from build123d import *

# Parameters (mm, degrees)
ESQUISSE1_W             = 30.5
ESQUISSE1_H             = 30.5
BOSS_EXTRU_1_DEPTH      = 9.35
TROU_TARAUD_M31_D       = 2.5
TROU_TARAUD_M31_DEPTH   = 8.5
TROU_TARAUD_M31_TIP     = 0.751075774
TROU_TARAUD_M32_D       = 2.5
TROU_TARAUD_M32_DEPTH   = 8.5
TROU_TARAUD_M32_TIP     = 0.751075774
PER_AGE1_AT_2_COUNT     = 2
PER_AGE1_AT_2_PITCH     = 24.890158698
ENL_V_MAT_EXTRU_3_DEPTH = 0.35
CHANFREIN1_SIZE         = 0.5


with BuildPart() as part:
    # Esquisse1 → Boss.-Extru.1 (new, symmetric)
    with BuildSketch(Plane.XY):
        Rectangle(ESQUISSE1_W, ESQUISSE1_H)
    extrude(amount=BOSS_EXTRU_1_DEPTH, both=True)

    # Esquisse2 → Révolution1 (revolve)
    with BuildSketch(Plane.XY, mode=Mode.PRIVATE) as r_volution1_sk:
        Polygon((35.05, 5.45), (35.05, 7.45), (20.55, 7.45), (20.55, 11.8), (15.25, 11.8), (15.25, 5.45), align=None)
    revolve(r_volution1_sk.sketch.rotate(Axis((15.25, 5.45, 0), (1, 0, 0)), 90), axis=Axis((15.25, 5.45, 0), (1, 0, 0)))

    # Esquisse3 → Révolution2 (revolve)
    with BuildSketch(Plane.XY):
        Polygon((-5.45, -35.05), (-7.45, -35.05), (-7.45, -20.55), (-11.8, -20.55), (-11.8, -15.25), (-5.45, -15.25), align=None)
    revolve(axis=Axis((-5.45, -15.25, 0), (0, -1, 0)))

    # Trou taraudé M31
    with Locations(Plane(origin=(15.25, 0, 0), x_dir=(0, 0, -1), z_dir=(1, 0, 0))):
        with Locations((0, -6.55)):
            Hole(TROU_TARAUD_M31_D / 2, depth=TROU_TARAUD_M31_DEPTH)
            with Locations((0, 0, -(TROU_TARAUD_M31_DEPTH + TROU_TARAUD_M31_TIP / 2))):  # 118° drill point
                Cone(0, TROU_TARAUD_M31_D / 2, TROU_TARAUD_M31_TIP, mode=Mode.SUBTRACT)

    # Trou taraudé M32
    with Locations(Plane(origin=(0, -15.25, 0), x_dir=(-1, 0, 0), z_dir=(0, -1, 0))):
        with Locations((-6.55, 0)):
            Hole(TROU_TARAUD_M32_D / 2, depth=TROU_TARAUD_M32_DEPTH)
            with Locations((0, 0, -(TROU_TARAUD_M32_DEPTH + TROU_TARAUD_M32_TIP / 2))):  # 118° drill point
                Cone(0, TROU_TARAUD_M32_D / 2, TROU_TARAUD_M32_TIP, mode=Mode.SUBTRACT)

    # Esquisse8 → Perçage1 (revolve, cut)
    with BuildSketch(Plane(origin=(-11.05, 11.05, -9.35), x_dir=(0, 1, 0), z_dir=(1, 0, 0))):
        Polygon((0, 0), (0, 19.811592145), (1.85, 18.7), (1.85, 5), (3.7, 5), (3.7, 0), align=None)
    per_age1 = revolve(axis=Axis((-11.05, 11.05, -20.660875039), (0, 0, 1)), mode=Mode.SUBTRACT)

    # Perçage1 at 2: Perçage1 ×2
    with Locations(*[Vector(0.7071067811865476, -0.7071067811865476, 0) * (i * PER_AGE1_AT_2_PITCH) for i in range(1, PER_AGE1_AT_2_COUNT)]):
        add(per_age1, mode=Mode.SUBTRACT)

    # Esquisse10 → Enlèv. mat.-Extru.3 (cut)
    with BuildSketch(Plane.XY.offset(-9.35)):
        with BuildLine():
            Line((15.25, 11.05), (-5.05, 11.05))
            ThreePointArc((-5.05, 11.05), (-6.807359313, 6.807359313), (-11.05, 5.05))
            Line((-11.05, 5.05), (-11.05, -15.25))
            Line((-11.05, -15.25), (0.55, -15.25))
            Line((0.55, -15.25), (0.55, -6.55))
            ThreePointArc((0.55, -6.55), (2.307359313, -2.307359313), (6.55, -0.55))
            Line((6.55, -0.55), (15.25, -0.55))
            Line((15.25, -0.55), (15.25, 11.05))
        make_face()
    enl_v_mat_extru_3 = extrude(amount=ENL_V_MAT_EXTRU_3_DEPTH, mode=Mode.SUBTRACT)

    # Symétrie1: Perçage1, Enlèv. mat.-Extru.3 across plane
    add(per_age1.mirror(Plane.XY), mode=Mode.SUBTRACT)
    add(enl_v_mat_extru_3.mirror(Plane.XY), mode=Mode.SUBTRACT)

    # Symétrie1 copy 1 sketch → Symétrie1 copy 1 (revolve, cut)
    with BuildSketch(Plane(origin=(6.55, -6.55, 9.35), x_dir=(0, 1, 0), z_dir=(1, 0, 0))):
        Polygon((0, 0), (0, -19.811592145), (1.85, -18.7), (1.85, -5), (3.7, -5), (3.7, 0), align=None)
    revolve(axis=Axis((6.55, -6.55, 20.660875039), (0, 0, 1)), mode=Mode.SUBTRACT)

    # Chanfrein1
    chanfrein1_edges = [part.edges().sort_by_distance(p)[0] for p in [
        (35.05, 5.45, -2),
        (20.55, 5.45, -6.35),
        (-3.45, -35.05, 0),
        (0.9, -20.55, 0),
        (15.25, -6.55, -1.25),
        (5.3, -15.25, 0),
        (15.25, -15.25, 0),
        (-15.25, -15.25, 0),
        (-15.25, 15.25, 0),
        (15.25, 15.25, 0),
    ]]
    chamfer(chanfrein1_edges, length=CHANFREIN1_SIZE)


solid = part.part
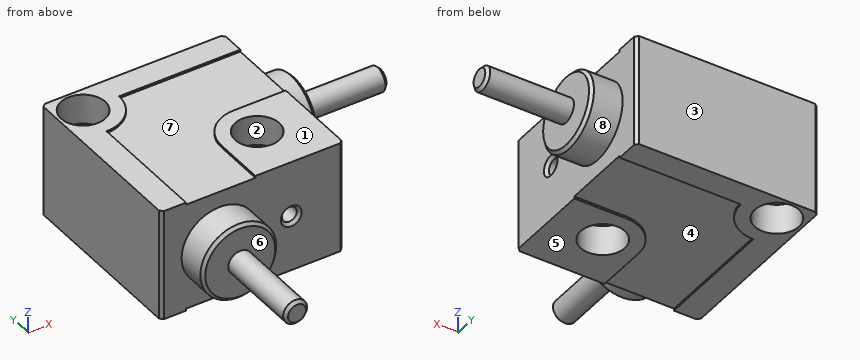
Read the model definition and answer for the solid it produces. Units are mm, in the model's axes. Face numbers are marked on the shaded views. A direction names the side the tool comes from. Coordinates: 2 decimals unless noted, no trailing zeros. Order: outer loops, then holes, each group sorted by start corner. A loop starts at its lowest first (then second) coordinate and runs counter-clockwise, first axis right, second up. Notation, with made-up numbers: M 88,33 L 121,33 A29 ccw 121,59 Z; hole C 66.25,51 d6. An arc over 180 degrees is marked long. Put each result on its own line as item: value. Start each with the question number.
Item 1: Section B-B, the plane x = 31.5 is taken. Determine the outline of the cut face in (y, z), plus the area to 3 significant figures.
Item 2: Given pin 1 Ø3.5 at (x, z) = (-8, -3) entering from -Y; pin 2 Ø6 at (x, y) = (6.55, -6.55) entering from -Z; pin 3 Ø8 at (x, y) = (-11, 10.5) entering from +Z; pin 4 Ø3 at (y, z) = (-20, 5.5) entering from -X, each flat-ended and moving along its own axis, determine where each tip first touches the part or whether it passes through.
Item 3: The mould has two halves that part along Y. Classify the marked faces 1, 2 and 3: +Y half, -Y half, draft (parallel to the pull), parting line (faces both ways), or undercut.
Item 4: Section C-C, the plane y = -23.5 is taken. Determine the outline of the cut face in (x, z), plus the area to 3 significant figures.
Item 5: Consider probe 1 along Y at (x, z) = (-11.05, -6.9); probe 2 along X at (y, z) = (-6.55, -2.5); probe 3 along Z at (x, y) = (12.25, -6.55). Determine where each line is inside the solid, lowest interval first. Write a range as [from, to].
Item 6: For the marked faces 4, 5, 6, 7 and 8, determine the directions among +Z, -Z, +X, -X, +Y, -Y from which every point of the face is accessible in a straight line to the end or side of a thin tool.
Item 7: Section A-A, the plane x = 9 is taken. Determine the outline of the cut face in (y, z).
Item 8: Section D-D, the plane z = -3 is taken. Count the separate pieces of the cut face and the enclosed holes in it, plus the area to 3 significant figures.
Computed:
1. outline: C 5.45,0 d4
1. area: 12.6 mm2
2. pin 1: stops at y = -20.55
2. pin 2: stops at z = -4.35
2. pin 3: stops at z = 9.35
2. pin 4: stops at x = -10.38
3. face 1: draft
3. face 2: undercut
3. face 3: +Y half
4. outline: C -5.45,0 d4
4. area: 12.6 mm2
5. probe 1: y = [-15.25, 7.35], [14.75, 15.25]
5. probe 2: x = [-15.25, 4.7], [8.4, 15.25]
5. probe 3: z = [-9.35, -1.25], [1.25, 9.35]
6. face 4: -Z
6. face 5: -Z, +X, -X, +Y, -Y
6. face 6: -Y
6. face 7: +Z
6. face 8: +X
7. outline: M -15.25,-9.35 L -9.32,-9.35 L -9.32,-4.35 L -3.78,-4.35 L -3.78,-9.35 L -0.55,-9.35 L -0.55,-9 L 11.05,-9 L 11.05,-9.35 L 15.25,-9.35 L 15.25,9.35 L 11.05,9.35 L 11.05,9 L -0.55,9 L -0.55,9.35 L -3.78,9.35 L -3.78,4.35 L -9.32,4.35 L -9.32,9.35 L -15.25,9.35 Z; hole C -6.55,0 d2.5
8. separate pieces: 1
8. enclosed holes: 2
8. area: 1,030 mm2
